The drawing under review shows one solid part. Ordinate dimensions are in mm from its lowest x, y, z. Coordinates: 2 decimals unless noted, no trailing zeros. Write each loop counter-clockwise with the first axis right and the second up, starting at its lowest first coordinate (ties: lowest second). Pieces come first, ordered by that corner, then holes.
Q1. For probe 1 along Y at (x, z) = (17.5, 0.35); probe 2 along X at (y, z) = (13.5, 2); probe 3 along X at (y, z) = (4, 0.25), list the stretches that pass through material, from the lowest coordinate up.
Q2. Take a section at C-C (x = 19). Give the boundary of the cut face in (y, z).
Q3. Take a section at B-B (y = 65). Give the boundary of the cut face in (x, z).
Q4. Take a section at A-A (x = 27). Give the boundary of the cut face in (y, z).
Q5. Take a section at D-D (z = 1.75). State how many separate pieces and enclosed holes the cut face has, and give its area (3 significant figures).
Q6. Insertion check: pin 1 (0.5 mm diameter, centred on x = 17.5, z = 2, fed in from -Y); pin 2 (0.9 mm diameter, centred on y = 84, z = 1, fed in from +X); pin 3 (0.9 mm diameter, centred on x = 11.5, z = 2, fed in from +Y). Each pin has a flat end and moves straight along its axis. Give the tip position at first contact, or say it passes through.
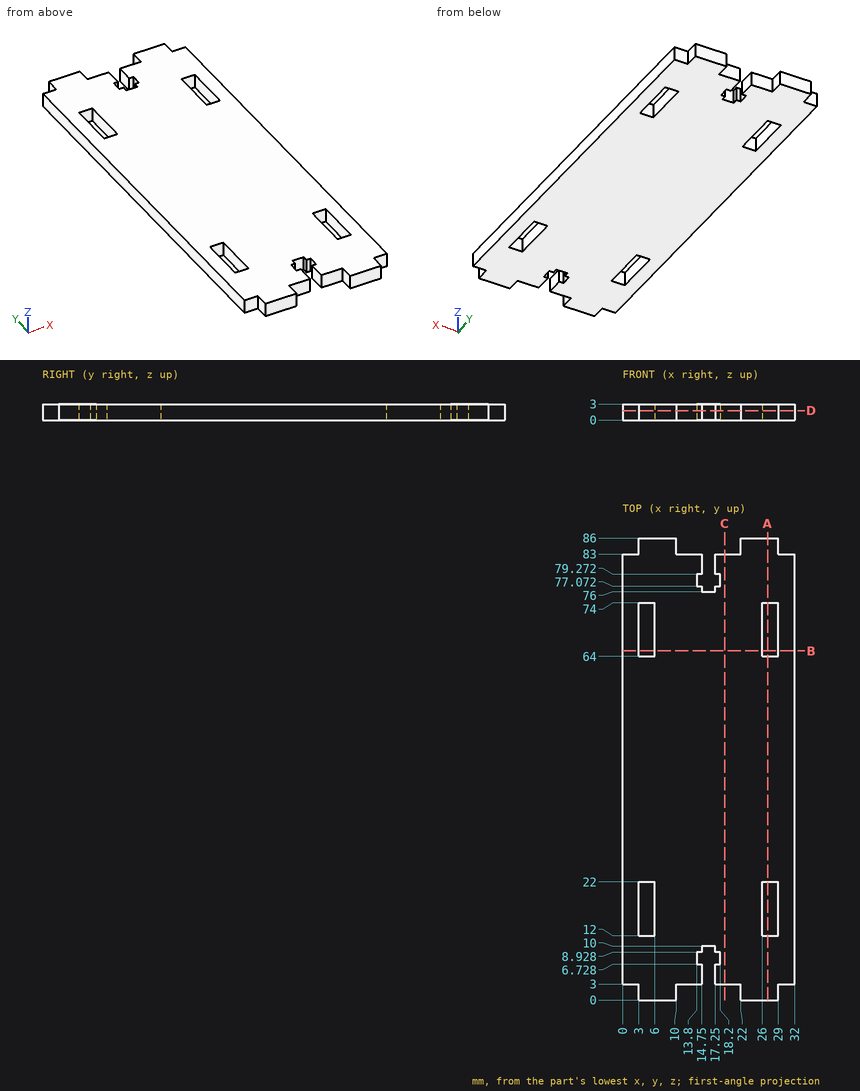
Response:
1. probe 1: y = 3 to 6.73, 8.93 to 77.07, 79.27 to 83
1. probe 2: x = 0 to 3, 6 to 26, 29 to 32
1. probe 3: x = 0 to 14.75, 17.25 to 32
2. outline: (3, 0) - (83, 0) - (83, 3) - (3, 3) - close
3. outline: (0, 0) - (3, 0) - (3, 3) - (0, 3) - close; (6, 0) - (26, 0) - (26, 3) - (6, 3) - close; (29, 0) - (32, 0) - (32, 3) - (29, 3) - close
4. outline: (0, 0) - (12, 0) - (12, 3) - (0, 3) - close; (22, 0) - (64, 0) - (64, 3) - (22, 3) - close; (74, 0) - (86, 0) - (86, 3) - (74, 3) - close
5. separate pieces: 1
5. enclosed holes: 4
5. area: 2,480 mm2
6. pin 1: stops at y = 3
6. pin 2: stops at x = 29
6. pin 3: stops at y = 83
